Source: CAD feature listing. Evaluate the final solid. Frame: model axes, mm. A direction names the side the tool comes from. Coordinates: 2 decimals unless noted, no trailing zeros. Loops run counter-clockwise (first coordinate to the right, second up) from the corner with the lowest first, then second, coordinate; pieces in that order, holes last. Notation, with made-up numbers: (17.25, -33) - (36.25, -33) arc R33 ccw to (36.25, 2) - close; hole circle Ø11 at (32, -31.5). An arc over 180 degrees is marked (long way). Use one line per item in the form item = value. Start each with the question number.
from build123d import *

# Parameters (mm, degrees)
IZIM1_W                     = 50
IZIM1_H                     = 50
IZIM1_H_2                   = 45
IZIM1_W_2                   = 45
Y_KSEKLIK_EKSTR_ZYON2_DEPTH = 4.5
IZIM2_R                     = 3
Y_KSEKLIK_EKSTR_ZYON3_DEPTH = 10
IZIM4_W                     = 15
IZIM4_H                     = 5
IZIM4_W_2                   = 5
IZIM4_H_2                   = 15
Y_KSEKLIK_EKSTR_ZYON5_DEPTH = 10
IZIM5_R                     = 2
KES_EKSTR_ZYON1_DEPTH       = 132.1
IZIM6_R                     = 2
KES_EKSTR_ZYON2_DEPTH       = 169.6


with BuildPart() as part:
    # Çizim1 → Yükseklik-Ekstrüzyon2 (new body)
    with BuildSketch(Plane.XY):
        Polygon((-35, -128.6), (-35, -116.312863708), (-52.209867178, -116.312863708), align=None)
        Polygon((-35, -116.312863708), (-148.890132822, -35), (-148.890132822, -47.287136292), (-52.209867178, -116.312863708), align=None)
        Polygon((-25, -35), (-35, -35), (-35, -116.312863708), (-35, -128.6), (35, -128.6), (35, -116.312863708), (35, -35), (25, -35), (25, -80), (25, -108.6), (-25, -108.6), (-25, -80), align=None)
        Polygon((-148.890132822, -47.287136292), (-166.1, -35), (-166.1, -128.6), (-35, -128.6), (-52.209867178, -116.312863708), (-148.890132822, -116.312863708), align=None)
        Polygon((-148.890132822, -35), (-166.1, -35), (-148.890132822, -47.287136292), align=None)
        Polygon((-35, 25), (-35, 35), (-148.890132822, 35), (-166.1, 35), (-166.1, -35), (-148.890132822, -35), (-35, -35), (-35, -25), (-80, -25), (-146.1, -25), (-146.1, 25), (-80, 25), align=None)
        Polygon((-25, 35), (-35, 35), (-35, 25), (-35, -25), (-35, -35), (-25, -35), (25, -35), (35, -35), (35, -25), (35, 25), (35, 35), (25, 35), align=None)
        Rectangle(IZIM1_W, IZIM1_H, mode=Mode.SUBTRACT)
        with Locations((0, -57.5)):
            Rectangle(IZIM1_W, IZIM1_H_2)
        Rectangle(IZIM1_W, IZIM1_H)
        with Locations((-57.5, 0)):
            Rectangle(IZIM1_W_2, IZIM1_H)
        with Locations((57.5, 0)):
            Rectangle(IZIM1_W_2, IZIM1_H)
        Polygon((148.890132822, 35), (35, 35), (35, 25), (80, 25), (146.1, 25), (146.1, -25), (80, -25), (35, -25), (35, -35), (148.890132822, -35), (166.1, -35), (166.1, 35), align=None)
        Polygon((148.890132822, -47.287136292), (148.890132822, -35), (35, -116.312863708), (52.209867178, -116.312863708), align=None)
        Polygon((148.890132822, -47.287136292), (166.1, -35), (148.890132822, -35), align=None)
        Polygon((166.1, -128.6), (166.1, -35), (148.890132822, -47.287136292), (148.890132822, -116.312863708), (52.209867178, -116.312863708), (35, -128.6), align=None)
        Polygon((52.209867178, -116.312863708), (35, -116.312863708), (35, -128.6), align=None)
        Polygon((52.209867178, 116.312863708), (35, 116.312863708), (148.890132822, 35), (148.890132822, 47.287136292), align=None)
        Polygon((148.890132822, 47.287136292), (148.890132822, 35), (166.1, 35), align=None)
        Polygon((166.1, 128.6), (35, 128.6), (52.209867178, 116.312863708), (148.890132822, 116.312863708), (148.890132822, 47.287136292), (166.1, 35), align=None)
        Polygon((52.209867178, 116.312863708), (35, 128.6), (35, 116.312863708), align=None)
        Polygon((35, 128.6), (-35, 128.6), (-35, 116.312863708), (-35, 35), (-25, 35), (-25, 80), (-25, 108.6), (25, 108.6), (25, 80), (25, 35), (35, 35), (35, 116.312863708), align=None)
        with Locations((0, 57.5)):
            Rectangle(IZIM1_W, IZIM1_H_2)
        Polygon((-35, 116.312863708), (-35, 128.6), (-52.209867178, 116.312863708), align=None)
        Polygon((-35, 116.312863708), (-52.209867178, 116.312863708), (-148.890132822, 47.287136292), (-148.890132822, 35), align=None)
        Polygon((-52.209867178, 116.312863708), (-35, 128.6), (-166.1, 128.6), (-166.1, 35), (-148.890132822, 47.287136292), (-148.890132822, 116.312863708), align=None)
        Polygon((-148.890132822, 35), (-148.890132822, 47.287136292), (-166.1, 35), align=None)
    extrude(amount=-Y_KSEKLIK_EKSTR_ZYON2_DEPTH)

    # Çizim2 → Yükseklik-Ekstrüzyon3 (add)
    with BuildSketch(Plane(origin=(0, 0, -4.5), x_dir=(-1, 0, 0), z_dir=(0, 0, -1))):
        Circle(IZIM2_R)
    extrude(amount=Y_KSEKLIK_EKSTR_ZYON3_DEPTH)

    # Çizim4 → Yükseklik-Ekstrüzyon5 (add)
    with BuildSketch(Plane(origin=(0, 0, -4.5), x_dir=(-1, 0, 0), z_dir=(0, 0, -1))):
        with Locations((-60, 0)):
            Rectangle(IZIM4_W, IZIM4_H)
        with Locations((0, -60)):
            Rectangle(IZIM4_W_2, IZIM4_H_2)
    extrude(amount=Y_KSEKLIK_EKSTR_ZYON5_DEPTH)

    # Çizim5 → Kes-Ekstrüzyon1 (cut, through all)
    with BuildSketch(Plane.XZ.offset(2.5)):
        with Locations((60, -9.5)):
            Circle(IZIM5_R)
        with Locations((60, -18.5)):
            Circle(IZIM5_R)
    extrude(amount=-KES_EKSTR_ZYON1_DEPTH, mode=Mode.SUBTRACT)

    # Çizim6 → Kes-Ekstrüzyon2 (cut, through all)
    with BuildSketch(Plane(origin=(2.5, 0, 0), x_dir=(0, 0, -1), z_dir=(1, 0, 0))):
        with Locations((9.5, -60)):
            Circle(IZIM6_R)
        with Locations((18.5, -60)):
            Circle(IZIM6_R)
    extrude(amount=-KES_EKSTR_ZYON2_DEPTH, mode=Mode.SUBTRACT)


solid = part.part
(1) Cut plane A-A, the plane x = 95. Output: boundary loops of the cut face in (y, z).
(2) Cut plane B-B, the plane y = 66. Output: boundary loops of the cut face in (x, z).
(3) Material intervals for line 1 (Y direction, x = -0.3, z = -9.5); line 2 (Y direction, x = -1, z = -9.5); line 3 (Z direction, x = 60, y = 1.4), sorted ascending.
(4) Cut plane C-C, the plane y = -31. Output: boundary loops of the cut face in (x, z), plus the area to 3 significant figures.
(5) Mould query, pull axis Y, two halves, no side actions, for faces 5 (the face through (-2.5, -62, -11)), 6 (the face through (101.227, 81.317, -2.218)), 7 (the face through (-92.74, 75.09, -2.22)), 8 (the face through (62, -2.5, -11)). Classes: +Y half, -Y half, draft (parallel to the pull), parting line (faces both ways), or undercut.
(6) Contact query for flat-ended pins moving along their axis: pin 1 (1.5 mm diameter, centred on y = -0.5, z = -8.5, fed in from +X); pin 2 (6 mm diameter, centred on x = -72.5, y = 20, fed in from -Z). Output: stop coordinate, or through.
(7) Access query for faces 1 (the face through (92.74, -75.09, -2.22)), 2 (the face through (2.5, -62, -11)), 3 (the face through (-39, 2, 0)), 4 (the face through (62, 2.5, -11)). Directions: +Z, -Z, +X, -X, +Y, -Y. A direction counts if a zero-diameter tool reaches every point of the face in a straight line with its end or side. Return the directions, or none.
Recorded:
q1.outline = (-128.6, -4.5) - (-116.31, -4.5) - (-116.31, 0) - (-128.6, 0) - close; (-85.76, -4.5) - (-73.48, -4.5) - (-73.48, 0) - (-85.76, 0) - close; (-35, -4.5) - (-25, -4.5) - (-25, 0) - (-35, 0) - close; (25, -4.5) - (35, -4.5) - (35, 0) - (25, 0) - close; (73.48, -4.5) - (85.76, -4.5) - (85.76, 0) - (73.48, 0) - close; (116.31, -4.5) - (128.6, -4.5) - (128.6, 0) - (116.31, 0) - close
q2.outline = (-166.1, -4.5) - (-148.89, -4.5) - (-148.89, 0) - (-166.1, 0) - close; (-122.68, -4.5) - (-105.47, -4.5) - (-105.47, 0) - (-122.68, 0) - close; (-35, -4.5) - (35, -4.5) - (35, 0) - (-35, 0) - close; (105.47, -4.5) - (122.68, -4.5) - (122.68, 0) - (105.47, 0) - close; (148.89, -4.5) - (166.1, -4.5) - (166.1, 0) - (148.89, 0) - close
q3.line_1 = -67.5 to -62, -58 to -52.5, -2.98 to 2.98
q3.line_2 = -67.5 to -62, -58 to -52.5, -2.83 to 2.83
q3.line_3 = -14.5 to -11.5, -7.5 to 0
q4.outline = (-166.1, -4.5) - (166.1, -4.5) - (166.1, 0) - (-166.1, 0) - close
q4.area = 1,490 mm²
q5.face_5 = draft
q5.face_6 = undercut
q5.face_7 = undercut
q5.face_8 = -Y half
q6.pin_1 = 67.5
q6.pin_2 = -4.5
q7.face_1 = +Z, -Z
q7.face_2 = -Z, +X, -Y
q7.face_3 = +Z, +X, -X, +Y, -Y
q7.face_4 = -Z, +X, +Y
